The model under review builds one solid part; all positions refer to its coordinate system, in mm. Face numbers are marked on the shaded views. A direction names the side the tool comes from. Coordinates: 2 decimals unless noted, no trailing zeros. Write each loop counter-clockwise with the first axis right and the second up, starting at its lowest first coordinate (ties: lowest second). Pieces come first, ordered by that corner, then holes.
```python
from build123d import *

# Parameters (mm, degrees)
SKETCH2_R               = 3.25
BOSS_EXTRUDE1_DEPTH     = 40
CUT_EXTRUDE1_DEPTH      = 81.126158627
CUT_EXTRUDE1_DEPTH_BACK = 81.126158627
SKETCH4_R               = 5
CUT_EXTRUDE2_DEPTH      = 50
SKETCH6_R               = 5
CUT_EXTRUDE4_DEPTH      = 50
SKETCH7_R               = 7.5
CUT_EXTRUDE5_DEPTH      = 3
CUT_EXTRUDE6_DEPTH      = 5.1
SKETCH5_R               = 7.5
CUT_EXTRUDE7_DEPTH      = 3


with BuildPart() as part:
    # Sketch2 → Boss-Extrude1 (new body)
    with BuildSketch(Plane(origin=(0, 0, 0), x_dir=(1, 0, 0), z_dir=(0, 1, 0))):
        with BuildLine():
            Line((-38.1, 0), (-38.1, 8))
            Line((-38.1, 8), (-9.67766953, 8))
            Line((-9.67766953, 8), (27.753941162, 45.431610691))
            ThreePointArc((27.753941162, 45.431610691), (45.431610691, 45.431610691), (45.431610691, 27.753941162))
            Line((45.431610691, 27.753941162), (8, -9.67766953))
            Line((8, -9.67766953), (8, -38.1))
            Line((8, -38.1), (0, -38.1))
            Line((0, -38.1), (0, 0))
            Line((0, 0), (-38.1, 0))
        make_face()
        with Locations(Location((18.738329701, 18.738329701, 0), (0, 0, 270))):
            Circle(SKETCH2_R, mode=Mode.SUBTRACT)
        with Locations(Location((36.592775926, 36.592775926, 0), (0, 0, 270))):
            Circle(SKETCH2_R, mode=Mode.SUBTRACT)
    extrude(amount=BOSS_EXTRUDE1_DEPTH)

    # Sketch3 → Cut-Extrude1 (cut, two sides: drawn at the far end of the back side and taken through both)
    with BuildSketch(Plane(origin=(0, 0, 0), x_dir=(0, -1, 0), z_dir=(0.7071067811865488, 0, 0.7071067811865464)).offset(-CUT_EXTRUDE1_DEPTH_BACK)):
        Polygon((-12.25, 9), (-27.75, 9), (-27.75, 69), (-35, 69), (-35, 89), (-5, 89), (-5, 69), (-12.25, 69), align=None)
    extrude(amount=CUT_EXTRUDE1_DEPTH + CUT_EXTRUDE1_DEPTH_BACK, mode=Mode.SUBTRACT)

    # Sketch4 → Cut-Extrude2 (cut)
    with BuildSketch(Plane.XY):
        with Locations((-19.05, 20)):
            Circle(SKETCH4_R)
    extrude(amount=-CUT_EXTRUDE2_DEPTH, mode=Mode.SUBTRACT)

    # Sketch6 → Cut-Extrude4 (cut)
    with BuildSketch(Plane.ZY):
        with Locations((19.05, 20)):
            Circle(SKETCH6_R)
    extrude(amount=-CUT_EXTRUDE4_DEPTH, mode=Mode.SUBTRACT)

    # Sketch7 → Cut-Extrude5 (cut)
    with BuildSketch(Plane(origin=(8, 0, 0), x_dir=(0, 0, -1), z_dir=(1, 0, 0))):
        with Locations((-19.05, 20)):
            Circle(SKETCH7_R)
    extrude(amount=-CUT_EXTRUDE5_DEPTH, mode=Mode.SUBTRACT)

    # Sketch10 → Cut-Extrude6 (cut)
    with BuildSketch(Plane(origin=(0, 0, 0), x_dir=(1, 0, 0), z_dir=(0, 1, 0))):
        Polygon((14.574197139, 22.902462264), (13.050018836, 17.214151399), (17.214151399, 13.050018836), (22.902462264, 14.574197139), (24.426640567, 20.262508004), (20.262508004, 24.426640567), align=None)
        Polygon((35.068597624, 30.904465061), (40.756908489, 32.428643364), (42.281086792, 38.116954229), (38.116954229, 42.281086792), (32.428643364, 40.756908489), (30.904465061, 35.068597624), align=None)
    extrude(amount=CUT_EXTRUDE6_DEPTH, mode=Mode.SUBTRACT)

    # Sketch5 → Cut-Extrude7 (cut)
    with BuildSketch(Plane(origin=(0, 0, -8), x_dir=(-1, 0, 0), z_dir=(0, 0, -1))):
        with Locations((19.05, 20)):
            Circle(SKETCH5_R)
    extrude(amount=-CUT_EXTRUDE7_DEPTH, mode=Mode.SUBTRACT)


solid = part.part
```
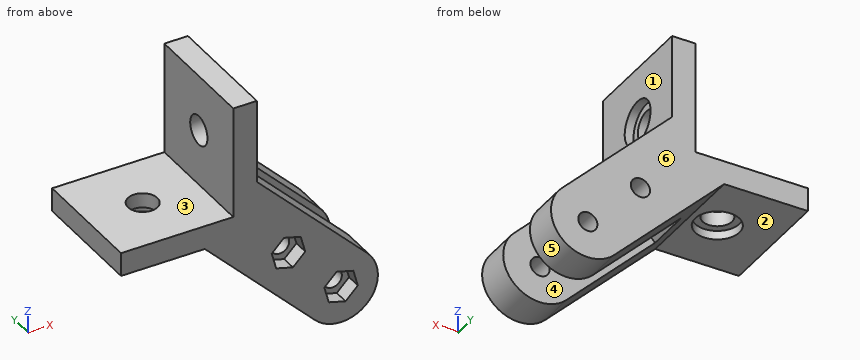
Item 1: For pin 1 (2 mm diameter, centred on y = 10, z = -24.5, fed in from +X); pin 2 (6 mm diameter, centred on y = 27.5, z = 15.5, fed in from -X); pin 3 (6 mm diameter, centred on x = 18.74, z = -18.74, fed in from -Y); pin 4 (5 mm diameter, centred on x = 13, y = 26, fed in from -Z), all flat-tipped, find the tip position at first contact; note any pin that passes through.
Solved:
pin 1: stops at x = 43.18
pin 2: stops at x = 0
pin 3: passes through
pin 4: stops at z = -32.46
Item 2: To check wall thickness, follow line 1 along Y through (x, z) = (2, 19); line 2 along Y through (x, z) = (30.5, -26.5); line 3 along Z through (x, y) = (-22, 13). State the ranges of each line that lie inside material, in increasing order.
Solved:
line 1: y = 0 to 15, 25 to 40
line 2: y = 0 to 12.25, 27.75 to 40
line 3: z = -8 to 0
Item 3: Take a section at A-A, the plane z = 19.05. Write out the cut boundary in (x, y).
Solved:
outline: (0, 0) - (8, 0) - (8, 12.5) - (5, 12.5) - (5, 15) - (0, 15) - close; (0, 25) - (5, 25) - (5, 27.5) - (8, 27.5) - (8, 40) - (0, 40) - close
Item 4: Take a section at B-B, the plane x = -19.05. Write out the cut boundary in (y, z).
Solved:
outline: (0, -8) - (12.5, -8) - (12.5, -5) - (15, -5) - (15, 0) - (0, 0) - close; (25, -5) - (27.5, -5) - (27.5, -8) - (40, -8) - (40, 0) - (25, 0) - close
Item 5: Take a section at C-C, the plane y = 20. Write out the cut boundary in (x, z).
Solved:
outline: (-38.1, -8) - (-26.55, -8) - (-26.55, -5) - (-24.05, -5) - (-24.05, 0) - (-38.1, 0) - close; (-14.05, -5) - (-11.55, -5) - (-11.55, -8) - (-9.68, -8) - (-2.47, -15.2) - (15.2, 2.47) - (8, 9.68) - (8, 11.55) - (5, 11.55) - (5, 14.05) - (0, 14.05) - (0, 0) - (-14.05, 0) - close; (0, 24.05) - (5, 24.05) - (5, 26.55) - (8, 26.55) - (8, 38.1) - (0, 38.1) - close
Item 6: Take a section at D-D, the plane y = 29. Write out the cut boundary in (x, z).
Solved:
outline: (-38.1, -8) - (-9.68, -8) - (27.75, -45.43) arc R12.5 ccw to (45.43, -27.75) - (8, 9.68) - (8, 38.1) - (0, 38.1) - (0, 0) - (-38.1, 0) - close; hole circle Ø6.5 at (18.74, -18.74); hole circle Ø6.5 at (36.59, -36.59)
Item 7: Mouldability with a two-part tool opening along Y and no side actions: class the marked faces 4, 5 and 6 as pulls with the +Y half, pulls with the -Y half, needs draft (parallel to the pull), parting line crosses it, or undercut.
Solved:
face 4: undercut
face 5: needs draft
face 6: pulls with the +Y half
Item 8: Machinability: for the marked faces 1, 2 and 3, which of the approach directions +Z, -Z, +X, -X, +Y, -Y give a long, thin tool a straight path to every point of the face, cutting with its end or side? Answer none if there is none.
Solved:
face 1: +Z, +X, +Y, -Y
face 2: -Z, -X, +Y, -Y
face 3: +Z, -X, +Y, -Y
